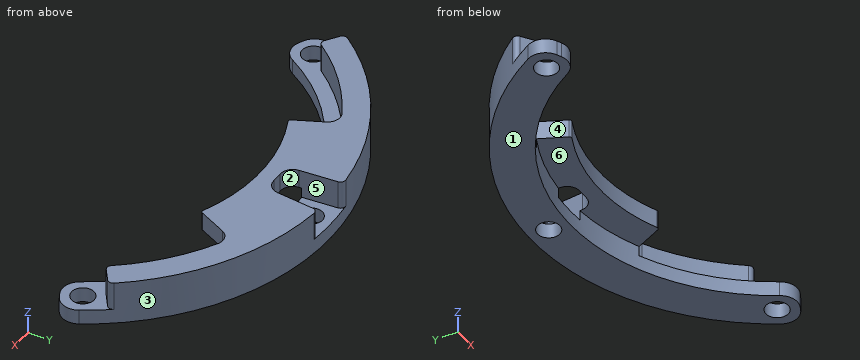
from build123d import *

# Parameters (mm, degrees)
EXTRUDE_1_DEPTH         = 3.699999999999999
EXTRUDE_2_DEPTH         = 2
EXTRUDE_3_DEPTH         = 2
EXTRUDE_4_DEPTH         = 2.9999999999999996
HOLE_WIZARD_4_5_4_5_1_D = 4.5
FILLET_1_R              = 0.5
FILLET_2_R              = 1
FILLET_3_R              = 2.5
FILLET_4_R              = 3.5


with BuildPart() as part:
    # 草图1 → 凸台-拉伸1 (new body)
    with BuildSketch(Plane.XY.offset(8.7)):
        with BuildLine():
            Line((14.79163916092453, 31.720772546282735), (18.637465342764905, 39.96817340831624))
            ThreePointArc((18.637465342764905, 39.96817340831624), (28.317533729903538, 33.807207566668026), (36.080540216984, 25.357535717230103))
            Line((36.080540216984, 25.357535717230103), (40.08948912998223, 28.17503968581122))
            ThreePointArc((40.08948912998223, 28.17503968581122), (24.49999999999949, 42.435244785437796), (4.3555555555549486, 48.80603585421044))
            Line((4.3555555555549486, 48.80603585421044), (3.3935020106793496, 38.025776205131926))
            ThreePointArc((3.3935020106793496, 38.025776205131926), (-2.3395e-13, 38.176897620148004), (-3.3935020106798226, 38.02577620513189))
            Line((-3.3935020106798226, 38.02577620513189), (-4.355555555555555, 48.80603585421038))
            ThreePointArc((-4.355555555555555, 48.80603585421038), (-24.50000000000001, 42.43524478543748), (-40.0894891299826, 28.17503968581074))
            Line((-40.0894891299826, 28.17503968581074), (-36.08054021698431, 25.357535717229652))
            ThreePointArc((-36.08054021698431, 25.357535717229652), (-28.317533729903744, 33.80720756666784), (-18.637465342764894, 39.96817340831625))
            Line((-18.637465342764894, 39.96817340831625), (-14.791639160924516, 31.720772546282742))
            ThreePointArc((-14.791639160924516, 31.720772546282742), (3.21e-15, 35.00000000000001), (14.79163916092453, 31.720772546282735))
        make_face()
    extrude(amount=-EXTRUDE_1_DEPTH)

    # 草图2 → 凸台-拉伸2 (add)
    with BuildSketch(Plane(origin=(0, 0, 5.000000000000001), x_dir=(-1, 0, 0), z_dir=(0, 0, -1))):
        with BuildLine():
            Line((-36.080540216984, 25.357535717230096), (-40.089489129982226, 28.175039685811218))
            ThreePointArc((-40.089489129982226, 28.175039685811218), (-24.499999999998106, 42.435244785438584), (-4.355555555551784, 48.806035854210705))
            Line((-4.355555555551784, 48.806035854210705), (-3.6533333333301714, 40.93730762465429))
            ThreePointArc((-3.6533333333301714, 40.93730762465429), (-10.67199534451459, 39.690282379527844), (-17.3696105575428, 37.249250047206296))
            Line((-17.3696105575428, 37.249250047206296), (-18.63746534276491, 39.96817340831625))
            ThreePointArc((-18.63746534276491, 39.96817340831625), (-28.317533729903555, 33.80720756666802), (-36.080540216984, 25.357535717230096))
        make_face()
    extrude(amount=EXTRUDE_2_DEPTH)

    # 草图3 → 凸台-拉伸3 (add)
    with BuildSketch(Plane(origin=(0, 0, 5.000000000000001), x_dir=(-1, 0, 0), z_dir=(0, 0, -1))):
        with BuildLine():
            Line((3.6533333333333347, 40.937307624654004), (4.355555555555555, 48.80603585421038))
            ThreePointArc((4.355555555555555, 48.80603585421038), (24.500000000000018, 42.43524478543748), (40.089489129982574, 28.175039685810727))
            Line((40.089489129982574, 28.175039685810727), (36.08054021698431, 25.357535717229652))
            ThreePointArc((36.08054021698431, 25.357535717229652), (28.317533729903737, 33.80720756666785), (18.637465342764894, 39.96817340831625))
            Line((18.637465342764894, 39.96817340831625), (17.369610557542792, 37.24925004720629))
            ThreePointArc((17.369610557542792, 37.24925004720629), (10.671995344516127, 39.69028237952743), (3.6533333333333347, 40.937307624654004))
        make_face()
    extrude(amount=EXTRUDE_3_DEPTH)

    # 草图4 → 凸台-拉伸4 (add)
    with BuildSketch(Plane.XY.offset(3)):
        with BuildLine():
            Line((-44.44504468553815, 20.63099616839955), (-37.27941503215546, 17.304774337167785))
            ThreePointArc((-37.27941503215546, 17.304774337167785), (-2.4282e-13, 41.099999999999994), (37.27941503215526, 17.304774337168233))
            Line((37.27941503215526, 17.304774337168233), (44.44504468553791, 20.630996168400085))
            ThreePointArc((44.44504468553791, 20.630996168400085), (-2.897e-13, 49.00000000000001), (-44.44504468553815, 20.63099616839955))
        make_face()
    extrude(amount=-EXTRUDE_4_DEPTH)

    # Ø4.5 (4.5) 直径孔1 (through all)
    with Locations(Plane.XY.offset(3)):
        with Locations((-38.97114317, 22.5), (38.97114317, 22.5), (0, 45)):
            Hole(HOLE_WIZARD_4_5_4_5_1_D / 2)

    # 圆角1
    fillet_1_edges = [part.edges().sort_by_distance(p)[0] for p in [
        (-14.791639160924518, 31.720772546282745, 6.85),
        (14.791639160924529, 31.72077254628274, 6.85),
    ]]
    fillet(fillet_1_edges, radius=FILLET_1_R)

    # 圆角2
    fillet_2_edges = [part.edges().sort_by_distance(p)[0] for p in [
        (-36.08054021698432, 25.357535717229656, 5.85),
        (-40.089489129982596, 28.175039685810734, 5.85),
        (-4.355555555555555, 48.80603585421038, 5.85),
        (4.3555555555533685, 48.80603585421058, 5.85),
        (40.08948912998223, 28.17503968581122, 5.85),
        (36.080540216984, 25.357535717230103, 5.85),
    ]]
    fillet(fillet_2_edges, radius=FILLET_2_R)

    # 圆角3
    fillet_3_edges = [part.edges().sort_by_distance(p)[0] for p in [
        (-18.637465342764898, 39.96817340831625, 5.85),
        (-3.3935020106798235, 38.02577620513189, 6.85),
        (3.3935020106793496, 38.02577620513193, 6.85),
        (18.637465342764905, 39.96817340831625, 5.85),
    ]]
    fillet(fillet_3_edges, radius=FILLET_3_R)

    # 圆角4
    fillet_4_edges = [part.edges().sort_by_distance(p)[0] for p in [
        (-44.44504468553815, 20.630996168399555, 1.5000000000000002),
        (44.44504468553791, 20.630996168400085, 1.5000000000000002),
        (37.27941503215526, 17.30477433716824, 1.5000000000000002),
        (-37.27941503215546, 17.304774337167785, 1.5000000000000002),
    ]]
    fillet(fillet_4_edges, radius=FILLET_4_R)


solid = part.part
Part model, mm, in its own coordinate system. Face numbers are marked on the shaded views. A direction names the side the tool comes from. Give positions to 0.01 mm unless a question says otherwise; leave off trailing zeros. Loops run counter-clockwise (first coordinate to the right, second up) from the corner with the lowest first, then second, coordinate; pieces in that order, holes last.
(1) Band-saw the part on D-D (x = -20). Write the cut outline in (y, z), and give its area (3 significant figures).
Return value:
outline: (35.91, 0) - (44.73, 0) - (44.73, 8.7) - (39.07, 8.7) - (39.07, 3) - (35.91, 3) - close
area: 58.8 mm2
(2) Band-saw the part on A-A (x = 0). Write the cut outline in (y, z), and give its area (3 significant figures).
Return value:
outline: (35, 5) - (38.18, 5) - (38.18, 8.7) - (35, 8.7) - close; (41.1, 0) - (42.75, 0) - (42.75, 3) - (41.1, 3) - close; (47.25, 0) - (49, 0) - (49, 3) - (47.25, 3) - close
area: 22.0 mm2
(3) Drill centre lines: line 1 along Z through (x, y) = (-13, 37); line 2 along Y through (x, z) = (19, 5.25); line 3 along Z through (x, y) = (-36, 25.5). Where is each one in solid material? Low to high.
Return value:
line 1: z = 5 to 8.7
line 2: y = 38.94 to 45.17
line 3: z = 0 to 3
(4) Band-saw the part on B-B (y = 22.5). Write the cut outline in (x, z).
Return value:
outline: (-43.17, 0) - (-41.22, 0) - (-41.22, 3) - (-43.17, 3) - close; (-36.72, 0) - (-34.39, 0) - (-34.39, 3) - (-36.72, 3) - close; (34.39, 0) - (36.72, 0) - (36.72, 3) - (34.39, 3) - close; (41.22, 0) - (43.17, 0) - (43.17, 3) - (41.22, 3) - close
(5) 3-axis set-ups, long thin cutter, end or side, ignore diameter. For the marked faces 4, 5 and 6: which of +Z, -Z, +X, -X, +Y, -Y reach the whole face in a straight line?
Return value:
face 4: +Z, -Y
face 5: +Z, +Y
face 6: -Z, -Y
(6) Pin check, flat tips, straight feed: pin 1 (6 mm diameter, centred on x = -32, y = 23.5, fed in from +Z); pin 2 (4.5 mm diameter, centred on x = -1, y = 36.5, fed in from -Z); pin 3 (3 mm diameter, centred on y = 31.5, z = 4, fed in from -X); pin 4 (4 mm diameter, centred on x = 38.97, y = 22.5, fed in from -Z). Stop position of each tip, or through.
Return value:
pin 1: stops at z = 3
pin 2: stops at z = 5
pin 3: stops at x = -38.74
pin 4: passes through
(7) Band-saw the part on C-C (y = 45). Write the cut outline in (x, z), and give its area (3 significant figures).
Return value:
outline: (-19.39, 0) - (-2.25, 0) - (-2.25, 3) - (-4.02, 3) - (-4.02, 8.7) - (-19.39, 8.7) - close; (2.25, 0) - (19.39, 0) - (19.39, 8.7) - (4.02, 8.7) - (4.02, 3) - (2.25, 3) - close
area: 278 mm2
(8) Pull direction X, two halves, no side cores. Call the marked faces 1, 2 and 3: pulls with the +X half, pulls with the -X half, needs draft (parallel to the pull), parting line crosses it, or undercut.
Return value:
face 1: needs draft
face 2: undercut
face 3: parting line crosses it
